```python
from build123d import *

# Parameters (mm, degrees)
EXTRUDE_1_DEPTH     = 20
CUT_EXTRUDE_START   = 3
SKETCH_2_W          = 25.638251078
SKETCH_2_H          = 25.026937626
CUT_EXTRUDE_1_DEPTH = 14


with BuildPart() as part:
    # 草图1 → 凸台-拉伸1 (new body)
    with BuildSketch(Plane.XY):
        Polygon((14, -7.5), (10, -7.5), (-7.5, 10), (-7.5, 14), (-14, 14), (-14, -14), (14, -14), align=None)
    extrude(amount=EXTRUDE_1_DEPTH)

    # 草图2 → 切除-拉伸1 (cut)
    with BuildSketch(Plane.XY.offset(CUT_EXTRUDE_START)):
        with Locations((2.819125539, 2.513468813)):
            Rectangle(SKETCH_2_W, SKETCH_2_H)
    extrude(amount=CUT_EXTRUDE_1_DEPTH, mode=Mode.SUBTRACT)


solid = part.part
```
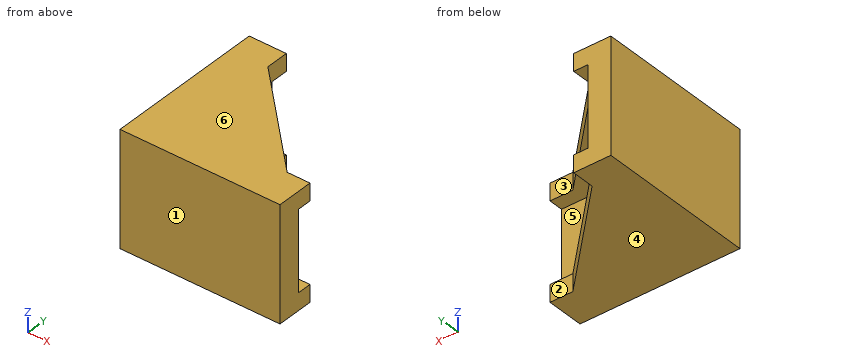
Geometry check sheet. Reference: the model listing, model coordinates, mm. Face numbers are marked on the shaded views. A direction names the side the tool comes from. Coordinates: 2 decimals unless noted, no trailing zeros. Order: outer loops, then holes, each group sorted by start corner. A loop starts at its lowest first (then second) coordinate and runs counter-clockwise, first axis right, second up. Notation, with made-up numbers: (58, -23.75) - (85, -23.75) arc R25 ccw to (85, -0.75) - close; hole circle Ø9 at (73, 3.25). An arc over 180 degrees is marked (long way). Answer in a Markdown table with one row per item. Add a question column.
1. Gauge pin test, flat ends, axial feed: pin 1 Ø1.5 at (x, z) = (12.5, 18.5) entering from +Y; pin 2 Ø5 at (x, z) = (1.5, 7.5) entering from +Y; pin 3 Ø4 at (y, z) = (9.5, 12.5) entering from +X. Record the tip position at first contact, or that the pin passes through.
2. Section check A-A (y = 4). Enter the section's corners in (x, z).
3. Section check C-C (z = 8.5). Enter the section's corners in (x, y), plus the area to 3 significant figures.
4. Access from +Z, -Z, +X, -X, +Y, -Y to the whole of each face (thin tool, end or side, straight path). Record for the marked faces 1 and 2.
5. Material ranges on L1, parallel to Z at x = -3.5, y = -6; L2, parallel to X at y = 4, z = 4, recorded low to high. Write a range as [from, to].
6. Draft check along Z on the marked faces 3, 4, 5 and 6. Enter one of: +Z half, -Z half, draft (parallel to the pull), parting line (faces both ways), or undercut.
7. Section check D-D (z = 1.75). Enter the section's corners in (x, y).
8. Section check B-B (x = 9.5). Enter the section's corners in (y, z).
Data:
| question | item | result |
|---|---|---|
| 1 | pin 1 | stops at y = -7.5 |
| 1 | pin 2 | stops at y = -10 |
| 1 | pin 3 | stops at x = -10 |
| 2 | outline | (-14, 0) - (-1.5, 0) - (-1.5, 3) - (-10, 3) - (-10, 17) - (-1.5, 17) - (-1.5, 20) - (-14, 20) - close |
| 3 | outline | (-14, -14) - (14, -14) - (14, -10) - (-10, -10) - (-10, 14) - (-14, 14) - close |
| 3 | area | 208 mm² |
| 4 | face 1 | +Z, -Z, +X, -X, -Y |
| 4 | face 2 | +Z, -Z, +X, +Y |
| 5 | L1 | z = [0, 3], [17, 20] |
| 5 | L2 | x = [-14, -10] |
| 6 | face 3 | draft |
| 6 | face 4 | -Z half |
| 6 | face 5 | undercut |
| 6 | face 6 | +Z half |
| 7 | outline | (-14, -14) - (14, -14) - (14, -7.5) - (10, -7.5) - (-7.5, 10) - (-7.5, 14) - (-14, 14) - close |
| 8 | outline | (-14, 0) - (-7, 0) - (-7, 3) - (-10, 3) - (-10, 17) - (-7, 17) - (-7, 20) - (-14, 20) - close |
